Input: part model. Units: mm. Frame: model coordinates. A direction names the side the tool comes from. Coordinates: 2 decimals unless noted, no trailing zeros. Write each loop counter-clockwise with the first axis right and the second up, starting at its lowest first coordinate (ties: lowest second). Pieces come first, ordered by that corner, then holes. Notation, with made-up numbers: (-13, -33) -> (43, -33) arc R10 ccw to (43, -18) -> close; hole circle Ø4 at (-26, -35.5). An arc over 180 degrees is marked (long way). Use one line per item in the form item = value. Start each with the question number.
(1) Cut plane B-B on x = -3. Return the cut outline in (y, z), plus the area to 3 significant figures.
(2) Set-up query: faces 1 (the face through (0, 0, -20)), 2 (the face through (-10.15, -0.41, -14.93)), 3 (the face through (-10.4, 0.1, -10)). Return all of +Z, -Z, +X, -X, +Y, -Y with unobstructed straight access to the full face (end or side cutting, diameter ignored); none if empty.
(3) First-contact query: pin 1 (1 mm diameter, centred on x = 13.5, z = 15.5, fed in from -Y); pin 2 (5 mm diameter, centred on x = 4.5, z = 12.5, fed in from +Y); pin 3 (3 mm diameter, centred on x = 16, y = 1, fed in from -Z). Flat tips, straight axial feed; report the tip coordinate or a pass-through.
(4) Cut plane D-D on x = 15.5. Return the cut outline in (y, z), plus the area to 3 significant figures.
(5) Cut plane A-A on y = 0. Return the cut outline in (x, z).
(6) Cut plane C-C on z = -6. Return the cut outline in (x, y), plus the area to 3 significant figures.
(7) Ray query, line 1 along Z through (x, y) = (13, 1.75); line 2 along Y through (x, z) = (4, 22.5); line 3 along X through (y, z) = (3, -16.5). Return the intervals inside material, ascending.
```python
from build123d import *

# Parameters (mm, degrees)
SKETCH1_W           = 40
SKETCH1_H           = 36.6
BOSS_EXTRUDE1_DEPTH = 10
SKETCH2_R           = 10.16
BOSS_EXTRUDE2_DEPTH = 10


with BuildPart() as part:
    # Sketch1 → Boss-Extrude1 (new, symmetric)
    with BuildSketch(Plane(origin=(0, 0, 0), x_dir=(1, 0, 0), z_dir=(0, 1, 0))):
        with Locations((8, -8.3)):
            Rectangle(SKETCH1_W, SKETCH1_H)
    extrude(amount=BOSS_EXTRUDE1_DEPTH, both=True)

    # Sketch2 → Boss-Extrude2 (add)
    with BuildSketch(Plane(origin=(0, 0, -10), x_dir=(-1, 0, 0), z_dir=(0, 0, -1))):
        with Locations(Location((0, 0, 0), (0, 0, 100.181748388))):
            Circle(SKETCH2_R)
    extrude(amount=BOSS_EXTRUDE2_DEPTH)


solid = part.part
```
Values:
q1.outline = (-10, -10) -> (-9.71, -10) -> (-9.71, -20) -> (9.71, -20) -> (9.71, -10) -> (10, -10) -> (10, 26.6) -> (-10, 26.6) -> close
q1.area = 926 mm2
q2.face_1 = -Z, +X, -X, +Y, -Y
q2.face_2 = -Z
q2.face_3 = -Z, -X
q3.pin_1 = -10
q3.pin_2 = 10
q3.pin_3 = -10
q4.outline = (-10, -10) -> (10, -10) -> (10, 26.6) -> (-10, 26.6) -> close
q4.area = 732 mm2
q5.outline = (-12, -10) -> (-10.16, -10) -> (-10.16, -20) -> (10.16, -20) -> (10.16, -10) -> (28, -10) -> (28, 26.6) -> (-12, 26.6) -> close
q6.outline = (-12, -10) -> (28, -10) -> (28, 10) -> (-12, 10) -> close
q6.area = 800 mm2
q7.line_1 = -10 to 26.6
q7.line_2 = -10 to 10
q7.line_3 = -9.71 to 9.71
